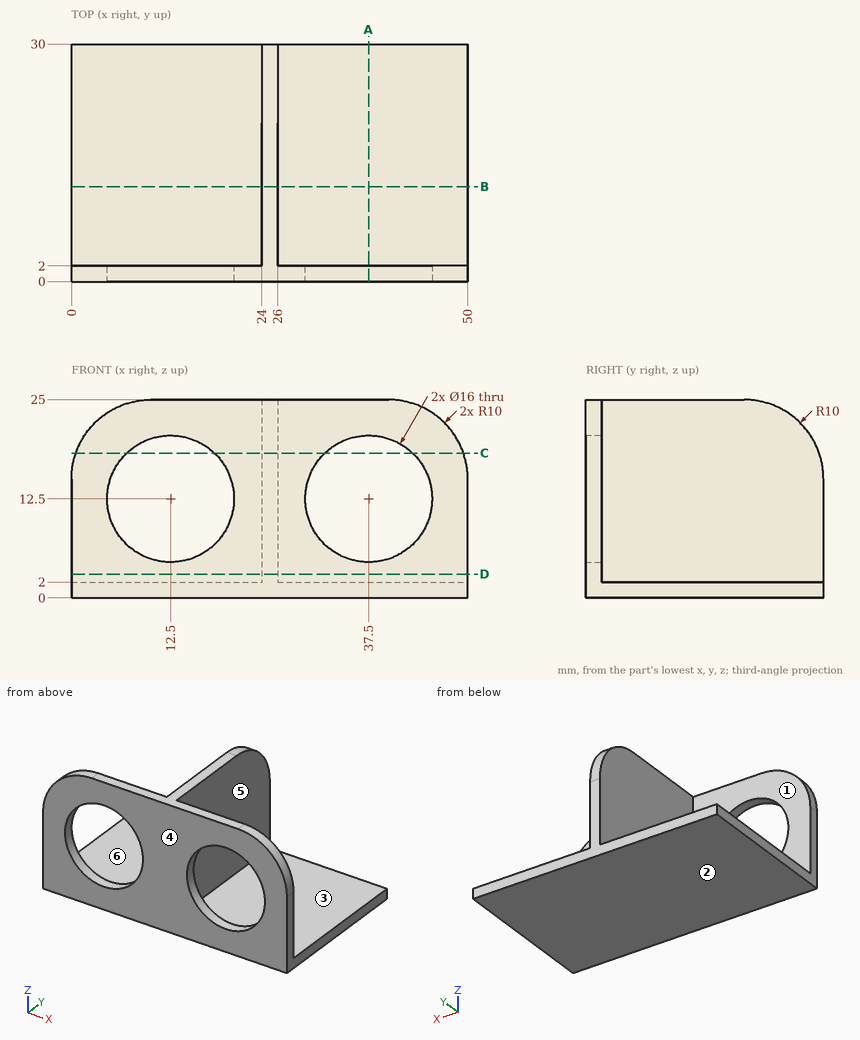
Could you check a few things on this drawing? It's one solid part, dimensions in mm from its lowest x, y, z. A direction names the side the tool comes from. Give positions to 0.01 mm unless a question says otherwise; leave off trailing zeros. Write each loop counter-clockwise with the first axis right and the second up, starting at its lowest first coordinate (ties: lowest second). Pieces come first, ordered by that corner, then holes.
(1) Will these pins go through, and if not, where does the flat tip stop? pin 1 (1 mm diameter, centred on x = 42.5, z = 5.5, fed in from +Y); pin 2 (5 mm diameter, centred on y = 18.5, z = 13.5, fed in from +X); pin 3 (7 mm diameter, centred on y = 21.5, z = 10.5, fed in from -X).
Output values:
pin 1: stops at y = 2
pin 2: stops at x = 26
pin 3: stops at x = 24
(2) Imagine slicing it at D-D, the plane z = 3. Write out the boundary of the cut face in (x, y).
Output values:
outline: (0, 0) - (50, 0) - (50, 2) - (26, 2) - (26, 30) - (24, 30) - (24, 2) - (0, 2) - close
(3) If I drill on L1, parallel to X at y = 1.5, z = 12.5; L2, parallel to Z at x = 12.5, y = 1.65; L3, parallel to Y at x = 22.5, z = 9.5, over which ranges is the centre line in solid material (lowest first)?
Output values:
L1: x = 0 to 4.5, 20.5 to 29.5, 45.5 to 50
L2: z = 0 to 4.5, 20.5 to 25
L3: y = 0 to 2
(4) Thinking about a two-plate mould opening in Z: for the marked faces 1, 2 and 3, which applies, pulls with the +Z half, pulls with the -Z half, needs draft (parallel to the pull), parting line crosses it, or undercut?
Output values:
face 1: needs draft
face 2: pulls with the -Z half
face 3: pulls with the +Z half
(5) Imagine slicing it at B-B, the plane y = 12. Write out the boundary of the cut face in (x, z).
Output values:
outline: (0, 0) - (50, 0) - (50, 2) - (26, 2) - (26, 25) - (24, 25) - (24, 2) - (0, 2) - close
(6) Imagine slicing it at A-A, the plane x = 37.5. Write out the boundary of the cut face in (y, z).
Output values:
outline: (0, 0) - (30, 0) - (30, 2) - (2, 2) - (2, 4.5) - (0, 4.5) - close; (0, 20.5) - (2, 20.5) - (2, 25) - (0, 25) - close
(7) Imagine slicing it at C-C, the plane z = 18.25. Write out the boundary of the cut face in (x, y), and give its area (3 significant figures).
Output values:
outline: (0.54, 0) - (6.94, 0) - (6.94, 2) - (0.54, 2) - close; (18.06, 0) - (31.94, 0) - (31.94, 2) - (26, 2) - (26, 29.46) - (24, 29.46) - (24, 2) - (18.06, 2) - close; (43.06, 0) - (49.46, 0) - (49.46, 2) - (43.06, 2) - close
area: 108 mm2
(8) On a 3-axis mill with a long thin cutter (end or side, diameter ignored), from which of +Z, -Z, +X, -X, +Y, -Y can I reach the whole of each face in a straight line? I mean the marked faces 4, 5 and 6. Say none if no direction works.
Output values:
face 4: +Z, -Z, +X, -X, -Y
face 5: +Z, +X, +Y
face 6: +Z, -X, +Y
